Can you work these out from the drawing? Everything is in mm from the part's minimum corner. A direction names the side the tool comes from. Coordinates: 2 decimals unless noted, no trailing zeros. Order: outer loops, then holes, each group sorted by start corner. A loop starts at its lowest first (then second) coordinate and runs counter-clockwise, first axis right, second up. Notation, with made-up numbers: (-25.75, 82) -> (-3.75, 82) arc R18 cw to (-3.75, 93) -> close; hole circle Ø1 at (-1, -33). An arc over 180 degrees is marked (long way). Use a Markdown table: item, result. Add a question column.
1) If we section it at C-C (x = 3.5): Write out the boundary of the cut face in (y, z).
2) Thinking about a two-plate mould opening in Y: for the marked faces 4, 5, 6 and 7, which applies, +Y half, -Y half, draft (parallel to the pull), parting line (faces both ways), or undercut?
3) If we section it at D-D (y = 7.75): Write out the boundary of the cut face in (x, z).
4) If we section it at A-A (z = 10): Write out the boundary of the cut face in (x, y).
5) If we section it at B-B (y = 5): Write out the boundary of the cut face in (x, z), plus the area to 3 significant figures.
6) If I drill on L1, parallel to Z at x = 4.75, y = 5; L2, parallel to Y at x = 5.6, z = 10; L3, parallel to X at y = 3, z = 5.5, over which ranges is the centre line in solid material (lowest first)? Write a range as [from, to].
7) Will these pins go through, and if not, where does the flat tip stop? pin 1 Ø1.5 at (x, y) = (1.5, 6) entering from -Z; pin 2 Ø0.8 at (x, y) = (1.5, 7) entering from +Z; pin 3 Ø5 at (y, z) = (7, 8) entering from +X.
8) Which directions (+Z, -Z, +X, -X, +Y, -Y) give clear straight access to the entire face, cutting with the end or side of a thin tool? Please do the marked faces 1, 2 and 3.
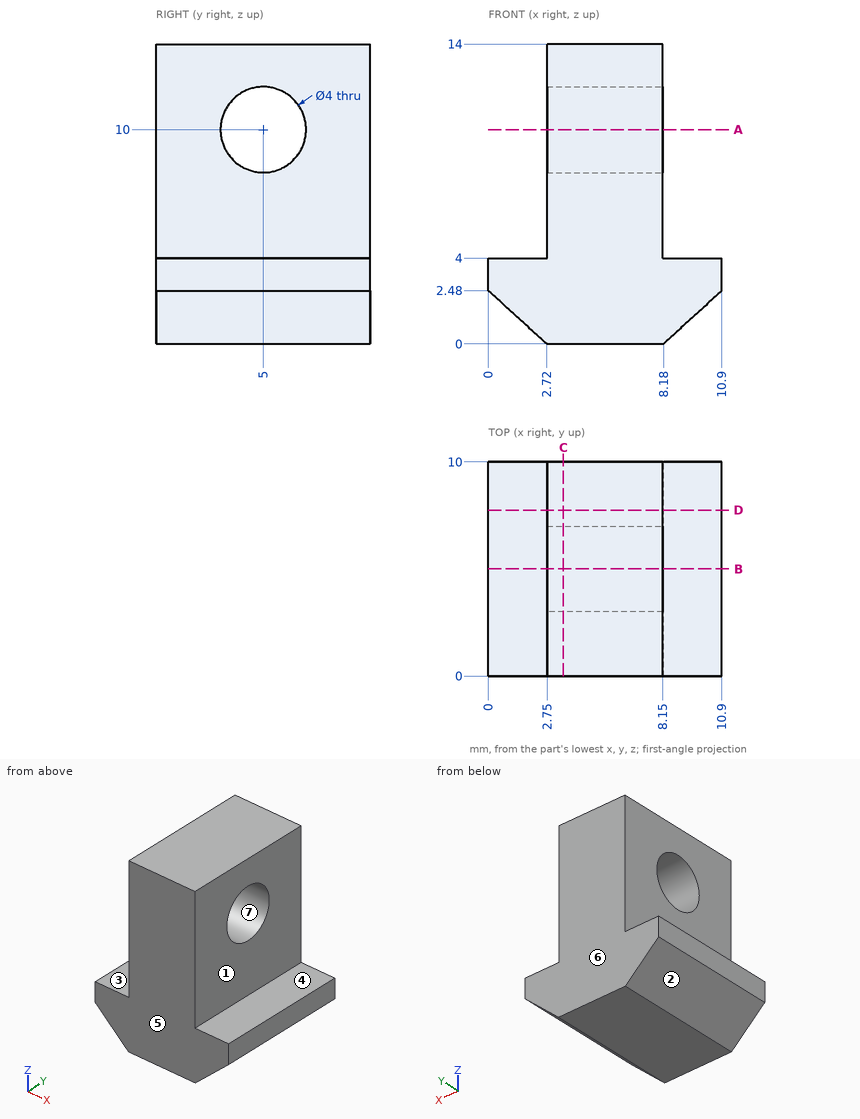
Answer sheet:
| question | item | result |
|---|---|---|
| 1 | outline | (0, 0) -> (10, 0) -> (10, 14) -> (0, 14) -> close; hole circle Ø4 at (5, 10) |
| 2 | face 4 | draft |
| 2 | face 5 | -Y half |
| 2 | face 6 | +Y half |
| 2 | face 7 | undercut |
| 3 | outline | (0, 2.48) -> (2.72, 0) -> (8.18, 0) -> (10.9, 2.48) -> (10.9, 4) -> (8.15, 4) -> (8.15, 14) -> (2.75, 14) -> (2.75, 4) -> (0, 4) -> close |
| 4 | outline | (2.75, 0) -> (8.15, 0) -> (8.15, 3) -> (2.75, 3) -> close; (2.75, 7) -> (8.15, 7) -> (8.15, 10) -> (2.75, 10) -> close |
| 5 | outline | (0, 2.48) -> (2.72, 0) -> (8.18, 0) -> (10.9, 2.48) -> (10.9, 4) -> (8.15, 4) -> (8.15, 8) -> (2.75, 8) -> (2.75, 4) -> (0, 4) -> close; (2.75, 12) -> (8.15, 12) -> (8.15, 14) -> (2.75, 14) -> close |
| 5 | area | 69.3 mm2 |
| 6 | L1 | [0, 8], [12, 14] |
| 6 | L2 | [0, 3], [7, 10] |
| 6 | L3 | [2.75, 8.15] |
| 7 | pin 1 | z = 0.43 |
| 7 | pin 2 | z = 4 |
| 7 | pin 3 | x = 8.15 |
| 8 | face 1 | +Z, +X, +Y, -Y |
| 8 | face 2 | -Z, -X, +Y, -Y |
| 8 | face 3 | +Z, -X, +Y, -Y |
